Could you check a few things on this model? Use its own coordinates, in mm. A direction names the side the tool comes from. Coordinates: 2 decimals unless noted, no trailing zeros. Loops run counter-clockwise (first coordinate to the right, second up) from the corner with the lowest first, then second, coordinate; pieces in that order, holes last.
1) Imagine slicing it at C-C on y = 0. Please give me the cut outline in (x, z), plus the area to 3 significant figures.
2) If I drill on line 1 along X through (y, z) = (9.8, -14.25); line 2 along Y through (x, z) = (11, -9); line 3 along Y through (x, z) = (3.25, 4), over which ranges is the centre line in solid material (lowest first)?
3) For faces 1 (the face through (1, 13.25, 10)), 2 (the face through (6, 0, 11.25)), 3 (the face through (11, 13.25, 10)), 4 (the face through (6, 11.75, 13)), 5 (the face through (4.6, 19.25, 3.6)), which set-ups out of +Z, -Z, +X, -X, +Y, -Y let a thin tool reach every point of the face, with its end or its side?
4) Imagine slicing it at A-A on z = 14.25. Please give me the cut outline in (x, y).
5) Will these pins go through, and if not, where does the flat tip stop? P1, Ø5.5, axis at x = 8.5, z = -13, coming from the +Y side; P2, Ø1, axis at x = 6.5, y = 14.5, coming from the -Z side; P3, Ø2.5, axis at x = 8.5, z = -13.5, coming from the -Y side; P4, Ø6.5, axis at x = 9, z = 8, coming from the +Y side.
6) Thinking about a two-plate mould opening in X: for faces 6 (the face through (6.3, 10.518, -13.296)), 7 (the face through (6, 9.25, -13)), 8 (the face through (5.779, 16.208, 11.246)), which applies, released by +X, released by -X, zero draft, split by the parting line, or undercut?
7) Imagine slicing it at B-B on x = 10.25. Please give me the cut outline in (y, z), plus the area to 3 significant figures.
8) Imagine slicing it at D-D on z = 8. Please give me the cut outline in (x, y), plus the area to 3 significant figures.
```python
from build123d import *

# Parameters (mm, degrees)
EXTRUDE_1_DEPTH     = 12
EXTRUDE_2_DEPTH     = 6
SKETCH_3_R          = 2
EXTRUDE_3_DEPTH     = 4
SKETCH_4_R          = 1
CUT_EXTRUDE_1_DEPTH = 30.138677046


with BuildPart() as part:
    # 草圖1 → 填料-伸長1 (new body)
    with BuildSketch(Plane(origin=(0, 0, 0), x_dir=(0, 0, -1), z_dir=(1, 0, 0))):
        Polygon((11.25, 11.75), (16.25, 11.75), (16.25, 9.25), (11.25, 9.25), (11.25, -9.25), (-11.25, -9.25), (-11.25, 9.25), (-16.25, 9.25), (-16.25, 11.75), (-11.25, 11.75), (-11.25, 13.25), (11.25, 13.25), align=None)
    extrude(amount=EXTRUDE_1_DEPTH)

    # 草圖2 → 填料-伸長2 (add)
    with BuildSketch(Plane(origin=(0, 13.25, 0), x_dir=(1, 0, 0), z_dir=(0, 1, 0))):
        with BuildLine():
            ThreePointArc((3.09526249, 0), (6, -11.25), (8.90473751, 0))
            ThreePointArc((8.90473751, 0), (6, 3.75), (3.09526249, 0))
        make_face()
    extrude(amount=EXTRUDE_2_DEPTH)

    # 草圖3 → 填料-伸長3 (add)
    with BuildSketch(Plane(origin=(0, 19.25, 0), x_dir=(1, 0, 0), z_dir=(0, 1, 0))):
        with Locations(Location((6, -5.25, 0), (0, 0, 270))):
            Circle(SKETCH_3_R)
    extrude(amount=EXTRUDE_3_DEPTH)

    # 草圖4 → 除料-伸長1 (cut, through all)
    with BuildSketch(Plane(origin=(0, 11.75, 0), x_dir=(1, 0, 0), z_dir=(0, 1, 0))):
        with Locations(Location((6, -14.25, 0), (0, 0, 270))):
            Circle(SKETCH_4_R)
        with Locations(Location((6, 14.25, 0), (0, 0, 270))):
            Circle(SKETCH_4_R)
    extrude(amount=-CUT_EXTRUDE_1_DEPTH, mode=Mode.SUBTRACT)


solid = part.part
```
Filled in:
1. outline: (0, -11.25) - (12, -11.25) - (12, 11.25) - (0, 11.25) - close
1. area: 270 mm2
2. line 1: x = 0 to 5, 7 to 12
2. line 2: y = -9.25 to 13.25
2. line 3: y = -9.25 to 19.25
3. face 1: +Z, -X, +Y
3. face 2: +Z, +X, -X, -Y
3. face 3: +Z, +X, +Y
3. face 4: +Z, +X, -X, +Y
3. face 5: +Y
4. outline: (0, 9.25) - (5, 9.25) - (5, 11.75) - (0, 11.75) - close; (7, 9.25) - (12, 9.25) - (12, 11.75) - (7, 11.75) - close
5. P1: stops at y = 13.25
5. P2: stops at z = -3.75
5. P3: stops at y = 9.25
5. P4: stops at y = 23.25
6. face 6: undercut
6. face 7: zero draft
6. face 8: split by the parting line
7. outline: (-9.25, -11.25) - (9.25, -11.25) - (9.25, -16.25) - (11.75, -16.25) - (11.75, -11.25) - (13.25, -11.25) - (13.25, 1.01) - (19.25, 1.01) - (19.25, 9.49) - (13.25, 9.49) - (13.25, 11.25) - (11.75, 11.25) - (11.75, 16.25) - (9.25, 16.25) - (9.25, 11.25) - (-9.25, 11.25) - close
7. area: 582 mm2
8. outline: (0, -9.25) - (12, -9.25) - (12, 13.25) - (11.33, 13.25) - (11.33, 19.25) - (0.67, 19.25) - (0.67, 13.25) - (0, 13.25) - close
8. area: 334 mm2
